Input: part model. Units: mm. Frame: model coordinates. Face numbers are marked on the shaded views. A direction names the side the tool comes from. Coordinates: 2 decimals unless noted, no trailing zeros. Loops run counter-clockwise (first coordinate to the right, second up) from the corner with the lowest first, then second, coordinate; pieces in that order, holes last.
Item 1: Reachability of the marked faces 1 and 2 from +Z, -Z, +X, -X, +Y, -Y: full face, straight path, thin tool, end or side. Return the list, or none.
Item 2: Section B-B on z = 17.4. Return loops of the section in (x, y), and give its area (3 significant figures).
Item 3: Pull-direction query (Z, two-part tool) for the marked faces 3, 4 and 5; classes: released by +Z, released by -Z, zero draft, split by the parting line, or undercut.
Item 4: Ray query, line 1 along X through (y, z) = (15, -29.09); line 2 along Z through (x, y) = (-37.5, 5.5); line 3 along Y through (x, z) = (-28.5, -3). Return the intervals inside material, ascending.
Item 5: Contact query for flat-ended pins moving along their axis: P1, Ø1.2, axis at x = -43, y = 14.5, coming from the +Z side; P2, Ø6, axis at y = 9, z = 16, coming from the +X side; P3, Ø5, axis at y = 20, z = -17.5, coming from the -X side. Output: stop coordinate, or through.
Item 6: Section A-A on y = 11.5. Give the number of separate pieces and of enclosed holes in the cut face, and give its area (3 significant figures).
Item 7: Section D-D on x = -38. Return loops of the section in (y, z).
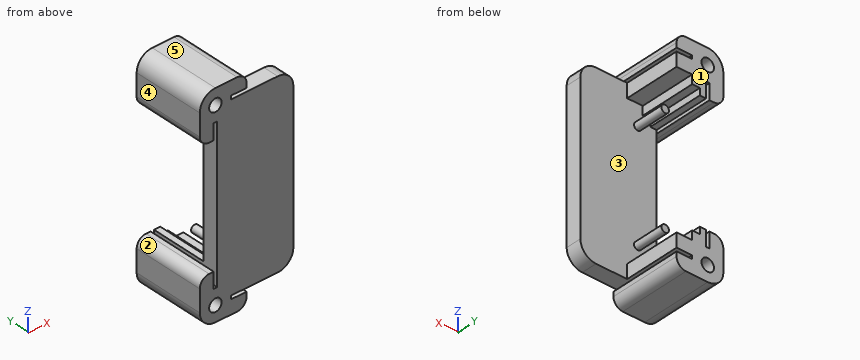
```python
from build123d import *

# Parameters (mm, degrees)
SKETCH1_W                  = 93.58
SKETCH1_H                  = 68.18
BASE_DEPTH                 = 5
SKETCH1_3_W                = 4.45
SKETCH1_3_H                = 4.45
SKETCH1_3_W_2              = 1.1
SKETCH1_3_H_2              = 1.1
SKETCH1_3_H_3              = 5
SKETCH1_3_W_3              = 5
WALLS_DEPTH                = 23
SKETCH1_4_W                = 63.58
SKETCH1_4_H                = 1.1
SKETCH1_4_W_2              = 5
SKETCH1_4_W_3              = 1.1
SKETCH1_4_H_2              = 5
SKETCH1_4_H_3              = 38.18
ACRYLIC_CUT_DEPTH          = 23
SKETCH2_W                  = 4.45
SKETCH2_H                  = 38.18
SKETCH2_W_2                = 63.58
SKETCH2_H_2                = 4.45
CUT_EXTRUDE2_DEPTH         = 63.293115189
SKETCH3_W                  = 58
SKETCH3_H                  = 42.5
BOARD_CUTOUT_DEPTH         = 18
SKETCH3_2_R                = 1.2
SCREW_HOLES_DEPTH          = 10
FILLET1_R                  = 5
FILLET3_R                  = 3
SKETCH6_R                  = 2
CUT_EXTRUDE3_DEPTH         = 63.293115189
BOTTOM_HALF_CUT_DEPTH      = 61.625342886
BOTTOM_HALF_CUT_DEPTH_BACK = 61.625342886
SKETCH5_W                  = 63.58
SKETCH5_H                  = 68.18
FILLET4_R                  = 5


with BuildPart() as part:
    # Sketch1 → Base (new body)
    with BuildSketch(Plane(origin=(0, 0, 0), x_dir=(1, 0, 0), z_dir=(0, 1, 0))):
        Rectangle(SKETCH1_W, SKETCH1_H)
    extrude(amount=BASE_DEPTH)

    # Sketch1<3> → Walls (add)
    with BuildSketch(Plane(origin=(0, 0, 0), x_dir=(1, 0, 0), z_dir=(0, 1, 0))):
        with Locations((-44.565, 31.865)):
            Rectangle(SKETCH1_3_W, SKETCH1_3_H)
        with Locations((-39.015, 31.865)):
            Rectangle(SKETCH1_3_W, SKETCH1_3_H)
        with Locations((-39.015, 26.315)):
            Rectangle(SKETCH1_3_W, SKETCH1_3_H)
        with Locations((-44.565, 26.315)):
            Rectangle(SKETCH1_3_W, SKETCH1_3_H)
        with Locations((-41.79, 31.865)):
            Rectangle(SKETCH1_3_W_2, SKETCH1_3_H)
        with Locations((-39.015, 29.09)):
            Rectangle(SKETCH1_3_W, SKETCH1_3_H_2)
        with Locations((-44.565, 29.09)):
            Rectangle(SKETCH1_3_W, SKETCH1_3_H_2)
        with Locations((-41.79, 26.315)):
            Rectangle(SKETCH1_3_W_2, SKETCH1_3_H)
        with Locations((-41.79, 29.09)):
            Rectangle(SKETCH1_3_W_2, SKETCH1_3_H_2)
        with Locations((-39.015, 21.59)):
            Rectangle(SKETCH1_3_W, SKETCH1_3_H_3)
        with Locations((-44.565, 21.59)):
            Rectangle(SKETCH1_3_W, SKETCH1_3_H_3)
        with Locations((-34.29, 26.315)):
            Rectangle(SKETCH1_3_W_3, SKETCH1_3_H)
        with Locations((-34.29, 31.865)):
            Rectangle(SKETCH1_3_W_3, SKETCH1_3_H)
        with Locations((-44.565, -21.59)):
            Rectangle(SKETCH1_3_W, SKETCH1_3_H_3)
        with Locations((-39.015, -21.59)):
            Rectangle(SKETCH1_3_W, SKETCH1_3_H_3)
        with Locations((-39.015, -26.315)):
            Rectangle(SKETCH1_3_W, SKETCH1_3_H)
        with Locations((-44.565, -26.315)):
            Rectangle(SKETCH1_3_W, SKETCH1_3_H)
        with Locations((-44.565, -31.865)):
            Rectangle(SKETCH1_3_W, SKETCH1_3_H)
        with Locations((-39.015, -31.865)):
            Rectangle(SKETCH1_3_W, SKETCH1_3_H)
        with Locations((-34.29, -31.865)):
            Rectangle(SKETCH1_3_W_3, SKETCH1_3_H)
        with Locations((-34.29, -26.315)):
            Rectangle(SKETCH1_3_W_3, SKETCH1_3_H)
        with Locations((-39.015, -29.09)):
            Rectangle(SKETCH1_3_W, SKETCH1_3_H_2)
        with Locations((-44.565, -29.09)):
            Rectangle(SKETCH1_3_W, SKETCH1_3_H_2)
        with Locations((-41.79, -31.865)):
            Rectangle(SKETCH1_3_W_2, SKETCH1_3_H)
        with Locations((-41.79, -29.09)):
            Rectangle(SKETCH1_3_W_2, SKETCH1_3_H_2)
        with Locations((-41.79, -26.315)):
            Rectangle(SKETCH1_3_W_2, SKETCH1_3_H)
        with Locations((34.29, -31.865)):
            Rectangle(SKETCH1_3_W_3, SKETCH1_3_H)
        with Locations((34.29, -26.315)):
            Rectangle(SKETCH1_3_W_3, SKETCH1_3_H)
        with Locations((39.015, -26.315)):
            Rectangle(SKETCH1_3_W, SKETCH1_3_H)
        with Locations((39.015, -31.865)):
            Rectangle(SKETCH1_3_W, SKETCH1_3_H)
        with Locations((44.565, -31.865)):
            Rectangle(SKETCH1_3_W, SKETCH1_3_H)
        with Locations((44.565, -26.315)):
            Rectangle(SKETCH1_3_W, SKETCH1_3_H)
        with Locations((39.015, -21.59)):
            Rectangle(SKETCH1_3_W, SKETCH1_3_H_3)
        with Locations((44.565, -21.59)):
            Rectangle(SKETCH1_3_W, SKETCH1_3_H_3)
        with Locations((41.79, -26.315)):
            Rectangle(SKETCH1_3_W_2, SKETCH1_3_H)
        with Locations((41.79, -29.09)):
            Rectangle(SKETCH1_3_W_2, SKETCH1_3_H_2)
        with Locations((41.79, -31.865)):
            Rectangle(SKETCH1_3_W_2, SKETCH1_3_H)
        with Locations((39.015, -29.09)):
            Rectangle(SKETCH1_3_W, SKETCH1_3_H_2)
        with Locations((44.565, -29.09)):
            Rectangle(SKETCH1_3_W, SKETCH1_3_H_2)
        with Locations((44.565, 21.59)):
            Rectangle(SKETCH1_3_W, SKETCH1_3_H_3)
        with Locations((34.29, 26.315)):
            Rectangle(SKETCH1_3_W_3, SKETCH1_3_H)
        with Locations((39.015, 21.59)):
            Rectangle(SKETCH1_3_W, SKETCH1_3_H_3)
        with Locations((34.29, 31.865)):
            Rectangle(SKETCH1_3_W_3, SKETCH1_3_H)
        with Locations((39.015, 26.315)):
            Rectangle(SKETCH1_3_W, SKETCH1_3_H)
        with Locations((39.015, 31.865)):
            Rectangle(SKETCH1_3_W, SKETCH1_3_H)
        with Locations((44.565, 31.865)):
            Rectangle(SKETCH1_3_W, SKETCH1_3_H)
        with Locations((44.565, 26.315)):
            Rectangle(SKETCH1_3_W, SKETCH1_3_H)
        with Locations((41.79, 26.315)):
            Rectangle(SKETCH1_3_W_2, SKETCH1_3_H)
        with Locations((41.79, 31.865)):
            Rectangle(SKETCH1_3_W_2, SKETCH1_3_H)
        with Locations((39.015, 29.09)):
            Rectangle(SKETCH1_3_W, SKETCH1_3_H_2)
        with Locations((41.79, 29.09)):
            Rectangle(SKETCH1_3_W_2, SKETCH1_3_H_2)
        with Locations((44.565, 29.09)):
            Rectangle(SKETCH1_3_W, SKETCH1_3_H_2)
        with Locations((-41.79, 21.59)):
            Rectangle(SKETCH1_3_W_2, SKETCH1_3_H_3)
        with Locations((-34.29, 29.09)):
            Rectangle(SKETCH1_3_W_3, SKETCH1_3_H_2)
        with Locations((-41.79, -21.59)):
            Rectangle(SKETCH1_3_W_2, SKETCH1_3_H_3)
        with Locations((-34.29, -29.09)):
            Rectangle(SKETCH1_3_W_3, SKETCH1_3_H_2)
        with Locations((34.29, -29.09)):
            Rectangle(SKETCH1_3_W_3, SKETCH1_3_H_2)
        with Locations((41.79, -21.59)):
            Rectangle(SKETCH1_3_W_2, SKETCH1_3_H_3)
        with Locations((41.79, 21.59)):
            Rectangle(SKETCH1_3_W_2, SKETCH1_3_H_3)
        with Locations((34.29, 29.09)):
            Rectangle(SKETCH1_3_W_3, SKETCH1_3_H_2)
    extrude(amount=WALLS_DEPTH)

    # Sketch1<4> → Acrylic Cut (cut)
    with BuildSketch(Plane(origin=(0, 0, 0), x_dir=(1, 0, 0), z_dir=(0, 1, 0))):
        with Locations((0, -29.09)):
            Rectangle(SKETCH1_4_W, SKETCH1_4_H)
        with Locations((-34.29, -29.09)):
            Rectangle(SKETCH1_4_W_2, SKETCH1_4_H)
        with Locations((34.29, -29.09)):
            Rectangle(SKETCH1_4_W_2, SKETCH1_4_H)
        with Locations((-41.79, -21.59)):
            Rectangle(SKETCH1_4_W_3, SKETCH1_4_H_2)
        with Locations((-41.79, 0)):
            Rectangle(SKETCH1_4_W_3, SKETCH1_4_H_3)
        with Locations((-41.79, 21.59)):
            Rectangle(SKETCH1_4_W_3, SKETCH1_4_H_2)
        with Locations((0, 29.09)):
            Rectangle(SKETCH1_4_W, SKETCH1_4_H)
        with Locations((-34.29, 29.09)):
            Rectangle(SKETCH1_4_W_2, SKETCH1_4_H)
        with Locations((34.29, 29.09)):
            Rectangle(SKETCH1_4_W_2, SKETCH1_4_H)
        with Locations((41.79, 21.59)):
            Rectangle(SKETCH1_4_W_3, SKETCH1_4_H_2)
        with Locations((41.79, 0)):
            Rectangle(SKETCH1_4_W_3, SKETCH1_4_H_3)
        with Locations((41.79, -21.59)):
            Rectangle(SKETCH1_4_W_3, SKETCH1_4_H_2)
    extrude(amount=ACRYLIC_CUT_DEPTH, mode=Mode.SUBTRACT)

    # Sketch2 → Cut-Extrude2 (cut, through all)
    with BuildSketch(Plane(origin=(0, 23, 0), x_dir=(1, 0, 0), z_dir=(0, 1, 0))):
        with Locations((-44.565, 0)):
            Rectangle(SKETCH2_W, SKETCH2_H)
        with Locations((0, 31.865)):
            Rectangle(SKETCH2_W_2, SKETCH2_H_2)
        with Locations((44.565, 0)):
            Rectangle(SKETCH2_W, SKETCH2_H)
        with Locations((0, -31.865)):
            Rectangle(SKETCH2_W_2, SKETCH2_H_2)
    extrude(amount=-CUT_EXTRUDE2_DEPTH, mode=Mode.SUBTRACT)

    # Sketch3 → Board Cutout (cut)
    with BuildSketch(Plane(origin=(0, 5, 0), x_dir=(1, 0, 0), z_dir=(0, 1, 0))):
        with Locations((-10.24, 0)):
            Rectangle(SKETCH3_W, SKETCH3_H)
    extrude(amount=BOARD_CUTOUT_DEPTH, mode=Mode.SUBTRACT)

    # Sketch3<2> → Screw Holes (add)
    with BuildSketch(Plane(origin=(0, 5, 0), x_dir=(1, 0, 0), z_dir=(0, 1, 0))):
        with Locations(Location((-35.19, -17.4, 0), (0, 0, 90))):
            Circle(SKETCH3_2_R)
        with Locations(Location((14.71, -17.4, 0), (0, 0, 90))):
            Circle(SKETCH3_2_R)
        with Locations(Location((14.71, 17.4, 0), (0, 0, 90))):
            Circle(SKETCH3_2_R)
        with Locations(Location((-35.19, 17.4, 0), (0, 0, 90))):
            Circle(SKETCH3_2_R)
    extrude(amount=SCREW_HOLES_DEPTH)

    # Fillet1
    fillet1_edges = [part.edges().sort_by_distance(p)[0] for p in [
        (-46.79, 11.5, 34.09),
        (46.79, 11.5, 34.09),
        (46.79, 11.5, -34.09),
        (-46.79, 11.5, -34.09),
    ]]
    fillet(fillet1_edges, radius=FILLET1_R)

    # Fillet3
    fillet3_edges = [part.edges().sort_by_distance(p)[0] for p in [
        (46.79, 11.5, -19.09),
        (31.79, 11.5, -34.09),
        (-31.79, 11.5, -34.09),
        (-46.79, 11.5, -19.09),
        (-31.79, 11.5, 34.09),
        (-46.79, 11.5, 19.09),
        (46.79, 11.5, 19.09),
        (31.79, 11.5, 34.09),
    ]]
    fillet(fillet3_edges, radius=FILLET3_R)

    # Sketch6 → Cut-Extrude3 (cut, through all)
    with BuildSketch(Plane(origin=(0, 23, 0), x_dir=(1, 0, 0), z_dir=(0, 1, 0))):
        with Locations(Location((-41.79, 29.09, 0), (0, 0, 270))):
            Circle(SKETCH6_R)
        with Locations(Location((41.79, 29.09, 0), (0, 0, 90))):
            Circle(SKETCH6_R)
        with Locations(Location((41.79, -29.09, 0), (0, 0, 270))):
            Circle(SKETCH6_R)
        with Locations(Location((-41.79, -29.09, 0), (0, 0, 90))):
            Circle(SKETCH6_R)
    extrude(amount=-CUT_EXTRUDE3_DEPTH, mode=Mode.SUBTRACT)

    # Sketch5 → Bottom Half Cut (cut, two sides: drawn at the far end of the back side and taken through both)
    with BuildSketch(Plane(origin=(0, 5, 0), x_dir=(1, 0, 0), z_dir=(0, 1, 0)).offset(-BOTTOM_HALF_CUT_DEPTH_BACK)):
        with Locations((15, 0)):
            Rectangle(SKETCH5_W, SKETCH5_H)
    extrude(amount=BOTTOM_HALF_CUT_DEPTH + BOTTOM_HALF_CUT_DEPTH_BACK, mode=Mode.SUBTRACT)

    # Fillet4
    fillet4_edges = [part.edges().sort_by_distance(p)[0] for p in [
        (-16.79, 2.5, 28.54),
        (-16.79, 2.5, -28.54),
    ]]
    fillet(fillet4_edges, radius=FILLET4_R)


solid = part.part
```
Results found:
1. face 1: +Z, -Z, +X, -X, +Y
1. face 2: -X, +Y, -Y
2. outline: (-41.24, 0) - (-16.79, 0) - (-16.79, 5) - (-33.99, 5) - (-33.99, 15) - (-36.39, 15) - (-36.39, 5) - (-41.24, 5) - close
2. area: 146 mm2
3. face 3: undercut
3. face 4: zero draft
3. face 5: released by +Z
4. line 1: x = -46.79 to -43.79, -39.79 to -36.79
4. line 2: z = -34.09 to -21.25, 21.25 to 34.09
4. line 3: y = 0 to 5
5. P1: stops at z = 34.05
5. P2: stops at x = -33.99
5. P3: stops at x = -45.94
6. separate pieces: 4
6. enclosed holes: 2
6. area: 333 mm2
7. outline: (0, -34.09) - (23, -34.09) - (23, -21.25) - (5, -21.25) - (5, 21.25) - (23, 21.25) - (23, 34.09) - (0, 34.09) - close
